Geometry: final body of the model. Coordinates: model frame, mm. A direction names the side the tool comes from. Give positions to 0.01 mm unless a question says otherwise; leave off trailing zeros. Write each loop counter-clockwise with the first axis right and the second up, starting at its lowest first coordinate (ties: lowest second). Pieces come first, ordered by that corner, then holes. Notation, with made-up numbers: M 6.25,-10.75 L 42.25,-10.75 A23 cw 42.25,23.25 Z; hole C 28,-15 d2. An arc over 180 degrees is marked long. Use a Markdown table: item, result. Add a question column.
(1) Cut plane D-D (y = -19). Output: boundary loops of the cut face in (x, z), plus the area to 3 significant figures.
(2) Pin query (flat end, axial travel): pin 1 Ø10 at (x, z) = (195, 13) entering from -Y; pin 2 Ø10 at (x, z) = (137, 16.5) entering from +Y; pin 3 Ø18.5 at (x, y) = (134, -27) entering from +Z; pin 4 Ø6 at (x, y) = (185.5, -6) entering from +Z. Return the tip coordinate at first contact, or that it passes through.
(3) Reachability of faces 1 (the flat face through (142, -28, 17)), 2 (the flat face through (131, -8, 40)) from +Z, -Z, +X, -X, +Y, -Y: full face, straight path, thin tool, end or side. Return the list, or none.
(4) Cut plane A-A (x = 146). Output: boundary loops of the cut face in (y, z), plus the area to 3 significant figures.
(5) Material intervals for L1, parallel to Z at x = 139, y = -35.5; L2, parallel to Y at x = 160.5, z = 20.5; L3, parallel to X at y = -19.5, z = 3.5, sorted ascending.
(6) Cut plane C-C (z = 5). Output: boundary loops of the cut face in (x, y).
(7) Cut plane B-B (y = -8.5). Output: boundary loops of the cut face in (x, z).
```python
from build123d import *

# Parameters (mm, degrees)
BOSS_EXTRU_1_START      = 83.500046
BOSS_EXTRU_1_DEPTH      = 135.5
ENL_V_MAT_EXTRU_1_DEPTH = 41
ENL_V_MAT_EXTRU_2_DEPTH = 41


with BuildPart() as part:
    # Esquisse1 → Boss.-Extru.1 (new body)
    with BuildSketch(Plane(origin=(0, 0, 0), x_dir=(0, 0, -1), z_dir=(1, 0, 0)).offset(BOSS_EXTRU_1_START)):
        Polygon((0, 0), (-40, 0), (-40, -17), (-17, -17), (-17, -40), (0, -40), align=None)
    extrude(amount=BOSS_EXTRU_1_DEPTH)

    # Esquisse2 → Enlèv. mat.-Extru.1 (cut, through all)
    with BuildSketch(Plane(origin=(0, 0, 0), x_dir=(1, 0, 0), z_dir=(0, 1, 0))):
        Polygon((219.000046471, 0), (179.000046471, -40), (219.000046471, -40), align=None)
    extrude(amount=-ENL_V_MAT_EXTRU_1_DEPTH, mode=Mode.SUBTRACT)

    # Esquisse3 → Enlèv. mat.-Extru.2 (cut, through all)
    with BuildSketch(Plane(origin=(0, 0, 0), x_dir=(-1, 0, 0), z_dir=(0, 0, -1))):
        Polygon((-219.000046471, 0), (-179.000046471, -40), (-219.000046471, -40), align=None)
    extrude(amount=-ENL_V_MAT_EXTRU_2_DEPTH, mode=Mode.SUBTRACT)


solid = part.part
```
Answer list:
| question | item | result |
|---|---|---|
| 1 | outline | M 83.5,0 L 200,0 L 200,17 L 83.5,17 Z |
| 1 | area | 1,980 mm² |
| 2 | pin 1 | y = -29 |
| 2 | pin 2 | y = 0 |
| 2 | pin 3 | z = 17 |
| 2 | pin 4 | z = 36.5 |
| 3 | face 1 | +Z, +X, -X, -Y |
| 3 | face 2 | +Z, +X, -X, +Y, -Y |
| 4 | outline | M -40,0 L 0,0 L 0,40 L -17,40 L -17,17 L -40,17 Z |
| 4 | area | 1,070 mm² |
| 5 | L1 | 0 to 17 |
| 5 | L2 | -17 to 0 |
| 5 | L3 | 83.5 to 199.5 |
| 6 | outline | M 83.5,-40 L 179,-40 L 214,-5 L 214,0 L 83.5,0 Z |
| 7 | outline | M 83.5,0 L 210.5,0 L 210.5,8.5 L 179,40 L 83.5,40 Z |
